```python
from build123d import *

# Parameters (mm, degrees)
SKETCH_1_R          = 4
SKETCH_1_R_2        = 3
EXTRUDE_1_DEPTH     = 25
SKETCH_2_W          = 106.280509252
SKETCH_2_H          = 41.998888678
CUT_EXTRUDE_1_DEPTH = 9.5
CUT_EXTRUDE_2_DEPTH = 3


with BuildPart() as part:
    # 草图1 → 凸台-拉伸1 (new, symmetric)
    with BuildSketch(Plane.XY):
        with BuildLine():
            Line((-43.874821937, 10), (43.874821937, 10))
            ThreePointArc((43.874821937, 10), (0, -45), (-43.874821937, 10))
        make_face()
        with Locations((0, -32.69)):
            Circle(SKETCH_1_R, mode=Mode.SUBTRACT)
        Circle(SKETCH_1_R_2, mode=Mode.SUBTRACT)
    extrude(amount=EXTRUDE_1_DEPTH, both=True)

    # 草图2 → 切除-拉伸1 (cut, symmetric)
    with BuildSketch(Plane.XY):
        Rectangle(SKETCH_2_W, SKETCH_2_H)
    extrude(amount=CUT_EXTRUDE_1_DEPTH, both=True, mode=Mode.SUBTRACT)

    # 草图3 → 切除-拉伸2 (cut, symmetric)
    with BuildSketch(Plane.XY):
        with BuildLine():
            Line((-8.4, -32.69), (-8.4, -18.964049075))
            Line((-8.4, -18.964049075), (8.4, -18.964049075))
            Line((8.4, -18.964049075), (8.4, -32.69))
            ThreePointArc((8.4, -32.69), (0, -41.09), (-8.4, -32.69))
        make_face()
    extrude(amount=CUT_EXTRUDE_2_DEPTH, both=True, mode=Mode.SUBTRACT)


solid = part.part
```
Work out the finished part from the listing and answer in its coordinate system (mm). A direction names the side the tool comes from. Give positions to 0.01 mm unless a question says otherwise; leave off trailing zeros. Loops run counter-clockwise (first coordinate to the right, second up) from the corner with the lowest first, then second, coordinate; pieces in that order, holes last. Notation, with made-up numbers: (40, 18) -> (72, 18) arc R22 cw to (72, 29) -> close; hole circle Ø5 at (62.5, 75.5). An arc over 180 degrees is marked (long way). Write item = value, one per line. Start each with the question number.
(1) Given pin 1 Ø3 at (y, z) = (-28.5, 0.5) entering from +X; pin 2 Ø3 at (x, z) = (24.5, -7) entering from +Y; pin 3 Ø1 at (y, z) = (-38, 16.5) entering from +X, each flat-ended and moving along its own axis, determine where each tip first touches the part or whether it passes through.
(2) Which of the six approach directions +Z, -Z, +X, -X, +Y, -Y give full straight-line access (tool end or side, diameter ignored) to faces 1 (the flat face through (8.4, -27, 0)), 2 (the flat face through (-1, -5, 9.5)), 3 (the flat face through (-1, 10, 17))?
(3) Find section B-B on y = 6. Give the vertices of the cut face in (x, z), and give its area (3 significant figures).
(4) Find section C-C on z = -12.5. Give the vertices of the cut face in (x, y), and give its area (3 significant figures).
(5) Find the intervals of material crossed by probe 1 along X at (y, z) = (0, -21); probe 2 along Z at (x, y) = (-1, -16); probe 3 along Z at (x, y) = (1.5, -25), in increasing order. Write a range as from..to.
(6) The mould has two halves that part along Z. Classify faces 4 (the flat face through (-1, -5, -9.5)), 5 (the flat face through (1, -11, 25)), 6 (the cylindrical face through (3.815, -31.489, 13.846)), 7 (the flat face through (-8.4, -27, 0)): +Z half, -Z half, draft (parallel to the pull), parting line (faces both ways), or undercut.
(7) Find section A-A on x = 0. Give the vertices of the cut face in (y, z), and give its area (3 significant figures).
(8) Find section D-D on x = -17. Give the vertices of the cut face in (y, z).
From the geometry:
q1.pin_1 = 36
q1.pin_2 = -21
q1.pin_3 = 24.87
q2.face_1 = +Y
q2.face_2 = +X, -X, +Y
q2.face_3 = +Z, -Z, +X, -X, +Y
q3.outline = (-44.6, -25) -> (44.6, -25) -> (44.6, -9.5) -> (-44.6, -9.5) -> close; (-44.6, 9.5) -> (44.6, 9.5) -> (44.6, 25) -> (-44.6, 25) -> close
q3.area = 2,770 mm^2
q4.outline = (-43.87, 10) arc R45 ccw (long way) to (43.87, 10) -> close; hole circle Ø8 at (0, -32.69); hole circle Ø6 at (0, 0)
q4.area = 3,990 mm^2
q5.probe_1 = -45..-3, 3..45
q5.probe_2 = -25..-9.5, 9.5..25
q5.probe_3 = -25..-3, 3..25
q6.face_4 = undercut
q6.face_5 = +Z half
q6.face_6 = draft
q6.face_7 = undercut
q7.outline = (-45, -25) -> (-36.69, -25) -> (-36.69, -3) -> (-41.09, -3) -> (-41.09, 3) -> (-36.69, 3) -> (-36.69, 25) -> (-45, 25) -> close; (-28.69, -25) -> (-3, -25) -> (-3, -9.5) -> (-21, -9.5) -> (-21, -3) -> (-28.69, -3) -> close; (-28.69, 3) -> (-21, 3) -> (-21, 9.5) -> (-3, 9.5) -> (-3, 25) -> (-28.69, 25) -> close; (3, -25) -> (10, -25) -> (10, -9.5) -> (3, -9.5) -> close; (3, 9.5) -> (10, 9.5) -> (10, 25) -> (3, 25) -> close
q7.area = 1,500 mm^2
q8.outline = (-41.67, -25) -> (10, -25) -> (10, -9.5) -> (-21, -9.5) -> (-21, 9.5) -> (10, 9.5) -> (10, 25) -> (-41.67, 25) -> close
